Source: CAD feature listing. Evaluate the final solid. Frame: model axes, mm. Face numbers are marked on the shaded views. A direction names the side the tool comes from. Give positions to 0.01 mm unless a question says otherwise; leave off trailing zeros. Order: outer loops, then holes, each group sorted by start corner. A loop starts at its lowest first (then second) coordinate and runs counter-clockwise, first axis right, second up.
Autodesk Inventor part; units mm, degrees
ref_plane "YZ Plane" through (0, 0, 0) normal (1, 0, 0) x (0, 1, 0)
ref_plane "XZ Plane" through (0, 0, 0) normal (0, 1, 0) x (-1, 0, 0)
ref_plane "XY Plane" through (0, 0, 0) normal (0, 0, 1) x (1, 0, 0)
sketch "Sketch1" plane through (0, 0, 0) normal (0, 1, 0) x (-1, 0, 0)
  circle A0 centre (0, 0) radius 4.7625
  dimension "d0" = 9.525
extrude "Extrusion1" add sketch "Sketch1" along normal blind 27.1272
thread "Thread1"
sketch "Sketch2" plane through (0, 0, 0) normal (0, -1, 0) x (1, 0, 0)
  circle A0 centre (0, 0) radius 4.7625
extrude "Extrusion2" add sketch "Sketch2" along normal blind 16.5608
sketch "Sketch3" plane through (0, -16.5608, 0) normal (0, -1, 0) x (1, 0, 0)
  circle A0 centre (0, 0) radius 4.7625
  line L0 (-4.0988, -7.0993) -> (-8.1976, 0)
  line L1 (-8.1976, 0) -> (-4.0988, 7.0993)
  line L2 (-4.0988, 7.0993) -> (4.0988, 7.0993)
  line L3 (4.0988, 7.0993) -> (8.1976, 0)
  line L4 (8.1976, 0) -> (4.0988, -7.0993)
  line L5 (4.0988, -7.0993) -> (-4.0988, -7.0993)
  dimension "d9" = 14.1986
  dimension "d10" = 14.1986
extrude "Extrusion3" add sketch "Sketch3" along normal blind 5.969 contours A0 | L0 L1 L2 L3 L4 L5
properties part number "3 8t 1 1 2 bolt"
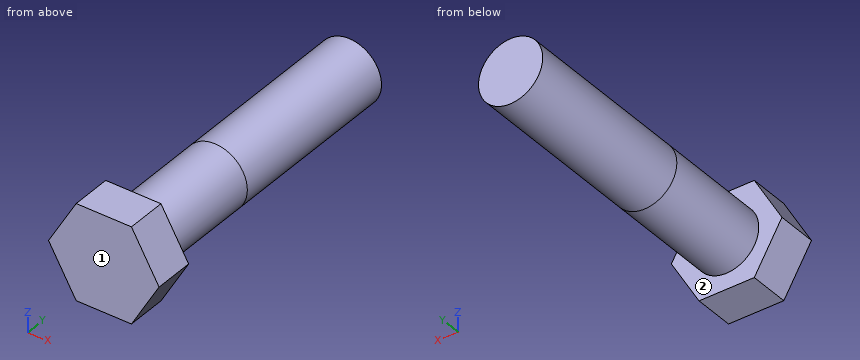
1) Reachability of the marked faces 1 and 2 from +Z, -Z, +X, -X, +Y, -Y: full face, straight path, thin tool, end or side. Return the list, or none.
Checks:
face 1: +Z, -Z, +X, -X, -Y
face 2: +Y
2) Section query B-B on z = -0.75. Output: boundary loops of the cut face in (x, y), and give its area (3 significant figures).
Checks:
outline: (-7.76, -22.53) - (7.76, -22.53) - (7.76, -16.56) - (4.7, -16.56) - (4.7, 27.13) - (-4.7, 27.13) - (-4.7, -16.56) - (-7.76, -16.56) - close
area: 504 mm2
3) Section query D-D on x = 5.25. Output: boundary loops of the cut face in (y, z), and give its area (3 significant figures).
Checks:
outline: (-22.53, -5.11) - (-16.56, -5.11) - (-16.56, 5.11) - (-22.53, 5.11) - close
area: 60.9 mm2
4) Section query C-C on y = 16. Output: boundary loops of the cut face in (x, z) (1 decimal).
Checks:
outline: circle Ø9.5 at (0, 0)
5) Section query A-A on x = 0. Output: boundary loops of the cut face in (y, z).
Checks:
outline: (-22.53, -7.1) - (-16.56, -7.1) - (-16.56, -4.76) - (27.13, -4.76) - (27.13, 4.76) - (-16.56, 4.76) - (-16.56, 7.1) - (-22.53, 7.1) - close
6) Ray query, L1, parallel to Y at x = -0.25, z = -5.75; L2, parallel to Z at x = 0, y = 6.5; L3, parallel to Z at x = 4.25, y = 1.5. Return the intervals inside material, ascending.
Checks:
L1: y = -22.53 to -16.56
L2: z = -4.76 to 4.76
L3: z = -2.15 to 2.15
7) First-contact query: pin 1 Ø8 at (y, z) = (-7, 3) entering from +X; pin 2 Ø6 at (x, y) = (1, -6.5) entering from +Z; pin 3 Ø8 at (y, z) = (9, -4.5) entering from -X. Flat tips, straight axial feed; report the tip coordinate or a pass-through.
Checks:
pin 1: stops at x = 4.76
pin 2: stops at z = 4.76
pin 3: stops at x = -4.74
